Autodesk Inventor part; units mm, degrees
ref_plane "YZ Plane" through (0, 0, 0) normal (1, 0, 0) x (0, 1, 0)
ref_plane "XZ Plane" through (0, 0, 0) normal (0, 1, 0) x (-1, 0, 0)
ref_plane "XY Plane" through (0, 0, 0) normal (0, 0, 1) x (1, 0, 0)
sketch "Boceto1" plane through (0, 0, 0) normal (0, 1, 0) x (-1, 0, 0)
  line L0 (27.5, 50) -> (-27.5, 50)
  line L1 (-27.5, 50) -> (-27.5, -50)
  line L2 (-27.5, -50) -> (27.5, -50)
  line L3 (27.5, -50) -> (27.5, 50)
  line L4 (27.5, 50) -> (-27.5, -50) construction
  line L5 (-27.5, 50) -> (27.5, -50) construction
  point P0 (0, 0)
  dimension "d0" = 55
  dimension "d1" = 100
extrude "Extrusión1" add sketch "Boceto1" along normal blind 30
sketch "Boceto3" plane through (-27.5, 0, 50) normal (0, 0, 1) x (1, 0, 0)
  circle A0 centre (27.5, 20) radius 5
  line L0 (0, 30) -> (55, 30)
  point P0 (27.5, 0)
  point P1 (27.5, 30)
  dimension "d10" = 10
  dimension "d11" = 10
extrude "Extrusión3" cut sketch "Boceto3" against normal blind 15
sketch "Boceto9" plane through (0, 0, 0) normal (0, -1, 0) x (1, 0, 0)
  line L0 (-37.5, 30) -> (37.5, 30)
  line L1 (37.5, 30) -> (37.5, -30)
  line L2 (37.5, -30) -> (-37.5, -30)
  line L3 (-37.5, -30) -> (-37.5, 30)
  line L4 (-37.5, 30) -> (37.5, -30) construction
  line L5 (37.5, 30) -> (-37.5, -30) construction
  point P0 (0, 0)
  dimension "d52" = 75
  dimension "d53" = 60
extrude "Extrusión7" add sketch "Boceto9" against normal blind 30
sketch "Boceto10" plane through (0, 30, 0) normal (0, 1, 0) x (1, 0, 0)
  line L0 (-32.5, 22.5) -> (32.5, 22.5)
  line L1 (32.5, 22.5) -> (32.5, -22.5)
  line L2 (32.5, -22.5) -> (-32.5, -22.5)
  line L3 (-32.5, -22.5) -> (-32.5, 22.5)
  line L4 (-32.5, 22.5) -> (32.5, -22.5) construction
  line L5 (32.5, 22.5) -> (-32.5, -22.5) construction
  point P0 (0, 0)
  dimension "d56" = 65
  dimension "d57" = 45
extrude "Extrusión8" cut sketch "Boceto10" against normal blind 20
properties part number "camera_support"
Geometry: final body of the model. Coordinates: model frame, mm. A direction names the side the tool comes from. Give positions to 0.01 mm unless a question says otherwise; leave off trailing zeros. Loops run counter-clockwise (first coordinate to the right, second up) from the corner with the lowest first, then second, coordinate; pieces in that order, holes last. Notation, with made-up numbers: (27.25, -20) - (81.25, -20) arc R12 cw to (81.25, -3) - close; hole circle Ø3 at (-20, 68). An arc over 180 degrees is marked (long way). One line per question, with ' | ' between items. Start each with the question number.
(1) Section query A-A on y = 20. Return loops of the section in (x, z), then the cut area to 4 significant figures.
(2) Section query C-C on z = -21. Return loops of the section in (x, y), then the cut area to 3 significant figures.
(3) Section query B-B on x = -30. Return loops of the section in (y, z).
(4) Pull-direction query (Y, two-part tool) for faces 6 (the flat face through (27.5, 15, -40)), 7 (the flat face through (-1, 30, 23)), 8 (the flat face through (0, 20, 35)); classes: released by +Y, released by -Y, zero draft, split by the parting line, or undercut.
(5) Reachability of faces 1 (the flat face through (33, 15, -30)), 2 (the flat face through (0, 10, 0)), 3 (the flat face through (-27.5, 15, -40)), 4 (the cylindrical face through (-1.08, 15.12, 42.6)), 5 (the flat face through (32, 15, 30)) from +Z, -Z, +X, -X, +Y, -Y: full face, straight path, thin tool, end or side. Return the list, or none.
(6) Section query D-D on y = 27. Return loops of the section in (x, z), then the cut area to 4 significant figures.
(7) Ray query, line 1 (X direction, y = 12.5, z = 0.5); line 2 (Z direction, x = -7, y = 15.25); line 3 (Y direction, x = 0, z = 46.5). Return the intervals inside material, ascending. Write a range as from..to.
(8) Contact query for flat-ended pins moving along their axis: pin 1 (3 mm diameter, centred on x = -0.5, y = 18.5, fed in from +Z); pin 2 (10 mm diameter, centred on x = 21, z = 10, fed in from +Y); pin 3 (3 mm diameter, centred on x = 33.5, y = 11, fed in from -Z). Output: stop coordinate, or through.
The answers:
1) outline: (-37.5, -30) - (-27.5, -30) - (-27.5, -50) - (27.5, -50) - (27.5, -30) - (37.5, -30) - (37.5, 30) - (27.5, 30) - (27.5, 50) - (5, 50) - (5, 35) - (-5, 35) - (-5, 50) - (-27.5, 50) - (-27.5, 30) - (-37.5, 30) - close; hole (-32.5, -22.5) - (32.5, -22.5) - (32.5, 22.5) - (-32.5, 22.5) - close | area: 3,625 mm2
2) outline: (-37.5, 0) - (37.5, 0) - (37.5, 30) - (32.5, 30) - (32.5, 10) - (-32.5, 10) - (-32.5, 30) - (-37.5, 30) - close | area: 950 mm2
3) outline: (0, -30) - (30, -30) - (30, -22.5) - (10, -22.5) - (10, 22.5) - (30, 22.5) - (30, 30) - (0, 30) - close
4) face 6: zero draft | face 7: released by +Y | face 8: undercut
5) face 1: -Z, +X, +Y, -Y | face 2: +Y | face 3: -Z, -X, +Y, -Y | face 4: +Z | face 5: +Z, +X, +Y, -Y
6) outline: (-37.5, -30) - (-27.5, -30) - (-27.5, -50) - (27.5, -50) - (27.5, -30) - (37.5, -30) - (37.5, 30) - (27.5, 30) - (27.5, 50) - (-27.5, 50) - (-27.5, 30) - (-37.5, 30) - close; hole (-32.5, -22.5) - (32.5, -22.5) - (32.5, 22.5) - (-32.5, 22.5) - close | area: 3,775 mm2
7) line 1: -37.5..-32.5, 32.5..37.5 | line 2: -50..-22.5, 22.5..50 | line 3: 0..15, 25..30
8) pin 1: z = 35 | pin 2: y = 10 | pin 3: z = -30
